from build123d import *

# Parameters (mm, degrees)
SKETCH1_R           = 2.65
BOSS_EXTRUDE1_DEPTH = 12.7
FILLET1_R           = 0.1


with BuildPart() as part:
    # Sketch1 → Boss-Extrude1 (new body)
    with BuildSketch(Plane(origin=(0, 0, 0), x_dir=(1, 0, 0), z_dir=(0, 1, 0))):
        with BuildLine():
            ThreePointArc((-48.121775191, 3.110386532), (-53.588631165, -7.404473703), (-43.07377093, -12.871329677))
            ThreePointArc((-43.07377093, -12.871329677), (-0.19527306, -6.260471572), (42.683224809, -12.871329677))
            ThreePointArc((42.683224809, -12.871329677), (53.198085044, -7.404473703), (47.73122907, 3.110386532))
            ThreePointArc((47.73122907, 3.110386532), (-0.19527306, 10.499528428), (-48.121775191, 3.110386532))
        make_face()
        with Locations(Location((-45.59777306, -4.880471572, 0), (0, 0, 270))):
            Circle(SKETCH1_R, mode=Mode.SUBTRACT)
        with Locations(Location((45.20722694, -4.880471572, 0), (0, 0, 270))):
            Circle(SKETCH1_R, mode=Mode.SUBTRACT)
    extrude(amount=BOSS_EXTRUDE1_DEPTH)

    # Fillet1
    fillet1_edges = [part.edges().sort_by_distance(p)[0] for p in [
        (45.20722694, 12.7, 2.230471572),
    ]]
    fillet(fillet1_edges, radius=FILLET1_R)


solid = part.part
The listing builds one solid part. Answer for the finished solid, in the listing's coordinates (mm). Give positions to 0.01 mm unless a question says otherwise; leave off trailing zeros. Write each loop counter-clockwise with the first axis right and the second up, starting at its lowest first coordinate (ties: lowest second). Pieces come first, ordered by that corner, then holes. Notation, with made-up numbers: (77.5, -1) - (136.5, -1) arc R18 ccw to (136.5, 9) - close; hole circle Ø4 at (35, 74). An arc over 180 degrees is marked (long way). Use a Markdown table: item, result.
1. Section D-D on z = -0.5 is taken. Write down the section's boundary in (x, y).
Values follow:
| item | result |
|---|---|
| outline | (-52.02, 0) - (51.63, 0) - (51.63, 12.7) - (-52.02, 12.7) - close |
2. For a pull along Z with two mould halves and no side action, classify faces 1 (the cylindrical face through (53.14, 6.26, 7.58)), 2 (the cylindrical face through (-48, 6, 6)), 3 (the flat face through (-1, 0, 1)) as released by +Z, released by -Z, zero draft, split by the parting line, or undercut.
Values follow:
| item | result |
|---|---|
| face 1 | split by the parting line |
| face 2 | undercut |
| face 3 | zero draft |
3. Each of these flat-tipped pins is pushed along its axis until it touches: P1, Ø3, axis at x = -27.5, z = -0.5, coming from the -Y side; P2, Ø2, axis at x = -20, y = 9.5, coming from the -Z side; P3, Ø5, axis at x = 1.5, y = 1.5, coming from the +Z side; P4, Ø2, axis at x = 29, y = 4, coming from the -Z side. Where does it stop, or does it pass through?
Values follow:
| item | result |
|---|---|
| P1 | stops at y = 0 |
| P2 | stops at z = -9.38 |
| P3 | stops at z = 6.32 |
| P4 | stops at z = -7.98 |
4. Section A-A on z = 4.5 is taken. Count the separate pieces of the cut face and the enclosed holes in it, plus the area to 3 significant figures.
Values follow:
| item | result |
|---|---|
| separate pieces | 3 |
| enclosed holes | 0 |
| area | 1,230 mm² |
5. Section B-B on y = 2.5 is taken. Write down the section's boundary in (x, z).
Values follow:
| item | result |
|---|---|
| outline | (-48.12, -3.11) arc R159.12 ccw to (47.73, -3.11) arc R8.38 ccw to (42.68, 12.87) arc R142.36 cw to (-43.07, 12.87) arc R8.38 ccw to start; hole circle Ø5.3 at (-45.6, 4.88); hole circle Ø5.3 at (45.21, 4.88) |
6. Section C-C on x = -33.5 is taken. Write down the section's boundary in (y, z).
Values follow:
| item | result |
|---|---|
| outline | (0, -6.98) - (12.7, -6.98) - (12.7, 10.21) - (0, 10.21) - close |
7. Find the intervals of material crossed by probe 1 along X at (y, z) = (8, 5); probe 2 along X at (y, z) = (4, 2.75); probe 3 along Z at (x, y) = (-1, 6.5), in increasing order. Write a range as from..to.
Values follow:
| item | result |
|---|---|
| probe 1 | x = -53.98..-48.25, -42.95..42.56, 47.85..53.59 |
| probe 2 | x = -53.7..-47.17, -44.02..43.63, 46.78..53.31 |
| probe 3 | z = -10.5..6.26 |
